from build123d import *

# Parameters (mm, degrees)
F0_W     = 180
F0_H     = 100
F2_DEPTH = 5
F3_D     = 5.5
F5_D     = 4.5
F7_D     = 4.4
F7_DEPTH = 12
F7_TIP   = 1.3218933619


with BuildPart() as f2:
    # F0 (on Top) → F2 (new body)
    with BuildSketch(Plane.XY):
        with Locations((39.8463645577, 50)):
            Rectangle(F0_W, F0_H)
    extrude(amount=-F2_DEPTH)

    # F3 (through all)
    with Locations(Plane.XY):
        with Locations((-140.1536354423, 95), (-40.1536354423, 95), (119.8463645577, 95), (219.8463645577, 95), (39.8463645577, 95)):
            Hole(F3_D / 2)

    # F5 (through all)
    with Locations(Plane(origin=(0, 0, -5), x_dir=(1, 0, 0), z_dir=(0, 0, -1))):
        with Locations((24.8463645577, -40), (54.8463645577, -40), (54.8463645577, -60), (24.8463645577, -60)):
            Hole(F5_D / 2)

    # F7
    with Locations(Plane.XY):
        with Locations((33.8463645577, 20), (45.8463645577, 20), (45.8463645577, 5), (33.8463645577, 5)):
            Hole(F7_D / 2, depth=F7_DEPTH)
            with Locations((0, 0, -(F7_DEPTH + F7_TIP / 2))):  # 118° drill point
                Cone(0, F7_D / 2, F7_TIP, mode=Mode.SUBTRACT)


solid = f2.part
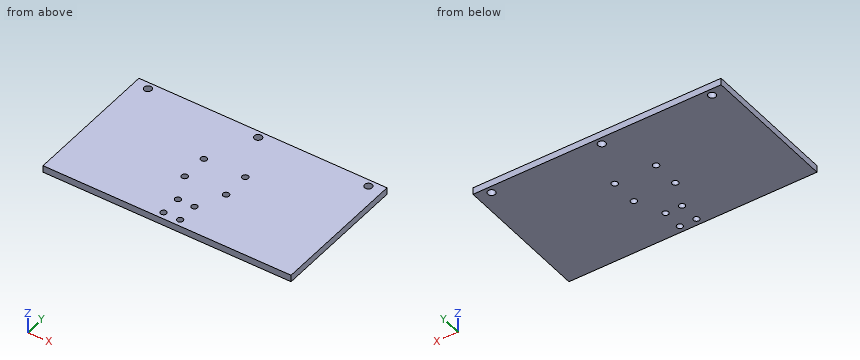
The listing builds one solid part. Answer for the finished solid, in the listing's coordinates (mm). Round coordinates to 2 decimals unless told otherwise and drop trailing zeros. Order: outer loops, then holes, each group sorted by start corner. A loop starts at its lowest first (then second) coordinate and runs counter-clockwise, first axis right, second up. Notation, with made-up numbers: (-7.5, 5.5) -> (41.5, 5.5) arc R19 cw to (41.5, 28.5) -> close; hole circle Ø4 at (78, 82.25). An arc over 180 degrees is marked (long way). One line per item, written item: value.
Item 1: Straight lines are drawn through the part: L1, parallel to X at y = 60, z = -1.85; L2, parallel to Y at x = -40.5, z = -3.35; L3, parallel to X at y = 38, z = -3.9. For each, find the intervals that lie inside material, in ascending order.
Taken from the geometry:
L1: x = -50.15 to 22.6, 27.1 to 52.6, 57.1 to 129.85
L2: y = 0 to 92.27, 97.73 to 100
L3: x = -50.15 to 23.82, 25.88 to 53.82, 55.88 to 129.85
Item 2: Find section B-B, the plane y = 95. Give the vertices of the cut face in (x, z).
Taken from the geometry:
outline: (-50.15, -5) -> (-42.9, -5) -> (-42.9, 0) -> (-50.15, 0) -> close; (-37.4, -5) -> (37.1, -5) -> (37.1, 0) -> (-37.4, 0) -> close; (42.6, -5) -> (117.1, -5) -> (117.1, 0) -> (42.6, 0) -> close; (122.6, -5) -> (129.85, -5) -> (129.85, 0) -> (122.6, 0) -> close
Item 3: Find section A-A, the plane y = 20. Give the vertices of the cut face in (x, z), then the cut area to 3 significant figures.
Taken from the geometry:
outline: (-50.15, -5) -> (31.65, -5) -> (31.65, 0) -> (-50.15, 0) -> close; (36.05, -5) -> (43.65, -5) -> (43.65, 0) -> (36.05, 0) -> close; (48.05, -5) -> (129.85, -5) -> (129.85, 0) -> (48.05, 0) -> close
area: 856 mm2
Item 4: Given P1, Ø3.5, axis at x = 45.85, y = 5, coming from the -Z side, flat-ended and moving along its own axis, determine where the tip first touches the part or whether it passes through.
Taken from the geometry:
P1: passes through
Item 5: Find section C-C, the plane y = 40. Give the vertices of the cut face in (x, z), then the cut area to 3 significant figures.
Taken from the geometry:
outline: (-50.15, -5) -> (22.6, -5) -> (22.6, 0) -> (-50.15, 0) -> close; (27.1, -5) -> (52.6, -5) -> (52.6, 0) -> (27.1, 0) -> close; (57.1, -5) -> (129.85, -5) -> (129.85, 0) -> (57.1, 0) -> close
area: 855 mm2
